from build123d import *

# Parameters (mm, degrees)
SKETCH1_R           = 3.25
BOSS_EXTRUDE1_DEPTH = 5


with BuildPart() as part:
    # Sketch1 → Boss-Extrude1 (new body)
    with BuildSketch(Plane.XY):
        with BuildLine():
            Line((-6.5, 75), (-6.5, 0))
            ThreePointArc((-6.5, 0), (0, -6.5), (6.5, 0))
            Line((6.5, 0), (6.5, 75))
            ThreePointArc((6.5, 75), (0, 81.5), (-6.5, 75))
        make_face()
        Circle(SKETCH1_R, mode=Mode.SUBTRACT)
        with BuildLine():
            Line((-3.25, 75), (-3.25, 45))
            ThreePointArc((-3.25, 45), (0, 41.75), (3.25, 45))
            Line((3.25, 45), (3.25, 75))
            ThreePointArc((3.25, 75), (0, 78.25), (-3.25, 75))
        make_face(mode=Mode.SUBTRACT)
        with BuildLine():
            Line((3.25, 35), (3.25, 25))
            ThreePointArc((3.25, 25), (0, 21.75), (-3.25, 25))
            Line((-3.25, 25), (-3.25, 35))
            ThreePointArc((-3.25, 35), (0, 38.25), (3.25, 35))
        make_face(mode=Mode.SUBTRACT)
    extrude(amount=BOSS_EXTRUDE1_DEPTH)


solid = part.part
Model file for the job. Use its own axes, mm. A direction names the side the tool comes from. Give positions to 0.01 mm unless a question says otherwise; leave off trailing zeros. Loops run counter-clockwise (first coordinate to the right, second up) from the corner with the lowest first, then second, coordinate; pieces in that order, holes last. Notation, with made-up numbers: (56.5, 1) -> (77.5, 1) arc R19 ccw to (77.5, 29) -> close; hole circle Ø3 at (72, -14.75). An arc over 180 degrees is marked (long way). Use a Markdown table: item, result. Add a question column.
(1) Slice it at A-A on y = 48. List the corners of the cut face in (x, z), and give its area (3 significant figures).
(2) Slice it at D-D on y = 24. List the corners of the cut face in (x, z), and give its area (3 significant figures).
(3) Wall check: line 1 along Y through (x, z) = (0, 2.8); line 2 along X through (y, z) = (68, 2.1); line 3 along Y through (x, z) = (3, 3.5). Give the ranges that are in metal, low to high.
(4) Slice it at B-B on x = 0. List the corners of the cut face in (y, z), and give its area (4 significant figures).
(5) Slice it at C-C on z = 2.7. List the corners of the cut face in (x, y).
(6) Tool access for faces 1 (the flat face through (-3.25, 60, 2)), 2 (the cylindrical face through (0.1, 81.5, 2.5)): list every direction of +Z, -Z, +X, -X, +Y, -Y with a clear straight run to the whole face (end or side of a thin tool).
Filled sheet:
| question | item | result |
|---|---|---|
| 1 | outline | (-6.5, 0) -> (-3.25, 0) -> (-3.25, 5) -> (-6.5, 5) -> close; (3.25, 0) -> (6.5, 0) -> (6.5, 5) -> (3.25, 5) -> close |
| 1 | area | 32.5 mm2 |
| 2 | outline | (-6.5, 0) -> (-3.09, 0) -> (-3.09, 5) -> (-6.5, 5) -> close; (3.09, 0) -> (6.5, 0) -> (6.5, 5) -> (3.09, 5) -> close |
| 2 | area | 34.1 mm2 |
| 3 | line 1 | -6.5 to -3.25, 3.25 to 21.75, 38.25 to 41.75, 78.25 to 81.5 |
| 3 | line 2 | -6.5 to -3.25, 3.25 to 6.5 |
| 3 | line 3 | -5.77 to -1.25, 1.25 to 23.75, 36.25 to 43.75, 76.25 to 80.77 |
| 4 | outline | (-6.5, 0) -> (-3.25, 0) -> (-3.25, 5) -> (-6.5, 5) -> close; (3.25, 0) -> (21.75, 0) -> (21.75, 5) -> (3.25, 5) -> close; (38.25, 0) -> (41.75, 0) -> (41.75, 5) -> (38.25, 5) -> close; (78.25, 0) -> (81.5, 0) -> (81.5, 5) -> (78.25, 5) -> close |
| 4 | area | 142.5 mm2 |
| 5 | outline | (-6.5, 0) arc R6.5 ccw to (6.5, 0) -> (6.5, 75) arc R6.5 ccw to (-6.5, 75) -> close; hole circle Ø6.5 at (0, 0); hole (-3.25, 25) arc R3.25 ccw to (3.25, 25) -> (3.25, 35) arc R3.25 ccw to (-3.25, 35) -> close; hole (-3.25, 45) arc R3.25 ccw to (3.25, 45) -> (3.25, 75) arc R3.25 ccw to (-3.25, 75) -> close |
| 6 | face 1 | +Z, -Z |
| 6 | face 2 | +Z, -Z, +Y |
